from build123d import *

# Parameters (mm, degrees)
F2_DEPTH = 9.525


# Not quite as in the source:
# - a variable given as a bare number and used for a length is read in inches; the dataset says mm whatever the document's units were


with BuildPart() as f2:
    # F1 (on Top) → F2 (new body)
    with BuildSketch(Plane.XY):
        with BuildLine():
            Line((4.1244459855, 7.14375), (4.1244459855, 35.71875))
            ThreePointArc((4.1244459855, 35.71875), (0, 38.1), (-4.1244459855, 35.71875))
            Line((-4.1244459855, 35.71875), (-4.1244459855, 7.14375))
            Line((-4.1244459855, 7.14375), (-8.248891971, 0))
            Line((-8.248891971, 0), (-32.9955678842, -14.2875))
            ThreePointArc((-32.9955678842, -14.2875), (-32.9955678842, -19.05), (-28.8711218987, -21.43125))
            Line((-28.8711218987, -21.43125), (-4.1244459855, -7.14375))
            Line((-4.1244459855, -7.14375), (4.1244459855, -7.14375))
            Line((4.1244459855, -7.14375), (28.8711218987, -21.43125))
            ThreePointArc((28.8711218987, -21.43125), (32.9955678842, -19.05), (32.9955678842, -14.2875))
            Line((32.9955678842, -14.2875), (8.248891971, 0))
            Line((8.248891971, 0), (4.1244459855, 7.14375))
        make_face()
        with BuildLine():
            ThreePointArc((2, 4.582575695), (4.1833001327, 2.7386127875), (5, 0))
            ThreePointArc((5, 0), (-2.7386127875, -4.1833001327), (-2, 4.582575695))
            Line((-2, 4.582575695), (-2, 7))
            Line((-2, 7), (2, 7))
            Line((2, 7), (2, 4.582575695))
        make_face(mode=Mode.SUBTRACT)
    extrude(amount=F2_DEPTH)


solid = f2.part
The model under review builds one solid part; all positions refer to its coordinate system, in mm. A direction names the side the tool comes from. Coordinates: 2 decimals unless noted, no trailing zeros. Loops run counter-clockwise (first coordinate to the right, second up) from the corner with the lowest first, then second, coordinate; pieces in that order, holes last. Notation, with made-up numbers: (62.5, 23.25) -> (74.5, 23.25) arc R33 cw to (74.5, 61.25) -> close; hole circle Ø11 at (-31.5, 71). An arc over 180 degrees is marked (long way). Use a Markdown table: item, result. Add a question column.
1. Add section C-C on y = 31. Write out the cut boundary in (x, z) (3 decimals).
2. Clearance check with flat-ended pins moving along their axes: pin 1 Ø3 at (x, z) = (0, 6.5) entering from -Y; pin 2 Ø1.2 at (y, z) = (6, 6) entering from -X; pin 3 Ø5 at (y, z) = (16.5, 3) entering from -X; pin 4 Ø3 at (x, y) = (0, 2) entering from +Z. State where each tip first meets the part, or that it passes through.
3. To check wall thickness, follow line 1 (Y direction, x = 0, z = 5.75); line 2 (X direction, y = 27, z = 9.25); line 3 (X direction, y = 6, z = 4.25). State the ranges of each line that lie inside material, in increasing order.
4. Add section D-D on x = 25. Write out the cut boundary in (y, z) (3 decimals).
5. Draft analysis for pull direction Y (two halves, no side actions). For faces 5 (the face through (0, 7, 5)), 6 (the face through (0.1, 38.1, 4.7)), 7 (the face through (-33.03, -18.99, 4.7)), state which applies: pulls with the +Y half, pulls with the -Y half, needs draft (parallel to the pull), parting line crosses it, or undercut.
6. Machinability: for faces 1 (the face through (-4.124, 22, 5)), 2 (the face through (2, 6, 5)), 3 (the face through (4.124, 21, 5)), 4 (the face through (0, -7.144, 5)), which of the approach directions +Z, -Z, +X, -X, +Y, -Y give a long, thin tool a straight path to every point of the face, cutting with its end or side? Answer none if there is none.
7. Add section B-B on z = 4. Write out the cut boundary in (x, y) (1 decimal).
8. Add section A-A on x = 0. Write out the cut boundary in (y, z) (3 decimals).
Returned:
| question | item | result |
|---|---|---|
| 1 | outline | (-4.124, 0) -> (4.124, 0) -> (4.124, 9.525) -> (-4.124, 9.525) -> close |
| 2 | pin 1 | stops at y = -7.14 |
| 2 | pin 2 | stops at x = -5.13 |
| 2 | pin 3 | stops at x = -4.12 |
| 2 | pin 4 | passes through |
| 3 | line 1 | y = -7.14 to -5, 7 to 38.1 |
| 3 | line 2 | x = -4.12 to 4.12 |
| 3 | line 3 | x = -4.78 to -2, 2 to 4.78 |
| 4 | outline | (-19.196, 0) -> (-9.671, 0) -> (-9.671, 9.525) -> (-19.196, 9.525) -> close |
| 5 | face 5 | undercut |
| 5 | face 6 | pulls with the +Y half |
| 5 | face 7 | parting line crosses it |
| 6 | face 1 | +Z, -Z, -X, +Y |
| 6 | face 2 | +Z, -Z |
| 6 | face 3 | +Z, -Z, +X, +Y |
| 6 | face 4 | +Z, -Z, -Y |
| 7 | outline | (-33, -14.3) arc R4.8 ccw to (-28.9, -21.4) -> (-4.1, -7.1) -> (4.1, -7.1) -> (28.9, -21.4) arc R4.8 ccw to (33, -14.3) -> (8.2, 0) -> (4.1, 7.1) -> (4.1, 35.7) arc R4.8 ccw to (-4.1, 35.7) -> (-4.1, 7.1) -> (-8.2, 0) -> close; hole (-2, 4.6) arc R5 ccw (long way) to (2, 4.6) -> (2, 7) -> (-2, 7) -> close |
| 8 | outline | (-7.144, 0) -> (-5, 0) -> (-5, 9.525) -> (-7.144, 9.525) -> close; (7, 0) -> (38.1, 0) -> (38.1, 9.525) -> (7, 9.525) -> close |
